Build history of the part. All positions in model axes, mm. A direction names the side the tool comes from. Give positions to 0.01 mm unless a question says otherwise; leave off trailing zeros. Return JSON: item names as keys, results as strings. Group by question number.
1) 3-axis set-ups, long thin cutter, end or side, ignore diameter. For faces 1 (the face through (-107.485, -173, 64)), 2 (the face through (-105.685, -173, 64)): which of +Z, -Z, +X, -X, +Y, -Y reach the whole face in a straight line?
2) Drop flat-ended pins along their axis: pin 1 (3 mm diameter, centred on y = -57, z = 57.5, fed in from +X); pin 2 (3 mm diameter, centred on y = -196, z = 73.5, fed in from +X); pin 3 (4.5 mm diameter, centred on y = -129, z = 53.5, fed in from +X). Give the stop position or say it passes through.
3) Slice it at A-A (y = -67.5). Count the separate pieces of the cut face and the enclosed holes in it, and give its area (3 significant figures).
4) Drill centre lines: probe 1 along Z at (x, y) = (-99, -293); probe 2 along Z at (x, y) = (-104.5, -229); probe 3 along X at (y, z) = (-174.5, 78.5). Where is each one in solid material? Low to high. Write a range as from..to.
5) Mould opens along X. For faces 3 (the face through (-87.485, -173, 64)), 4 (the face through (-102, -350, 69)), 5 (the face through (-89.285, -173, 64)) say: released by +X, released by -X, zero draft, split by the parting line, or undercut.
```python
from build123d import *

# Parameters (mm, degrees)
F0_R     = 2.5
F1_DEPTH = 350


with BuildPart() as f1:
    # F0 (on Front) → F1 (new body)
    with BuildSketch(Plane.XZ):
        with BuildLine():
            Line((-91.984542, 44.065978), (-88.984542, 44.065978))
            ThreePointArc((-88.984542, 44.065978), (-87.923881, 44.505318), (-87.484542, 45.565978))
            Line((-87.484542, 45.565978), (-87.484542, 48.565978))
            Line((-87.484542, 48.565978), (-87.484542, 50.465978))
            Line((-87.484542, 50.465978), (-87.784542, 50.465978))
            ThreePointArc((-87.784542, 50.465978), (-87.925963, 50.524557), (-87.984542, 50.665978))
            Line((-87.984542, 50.665978), (-87.984542, 50.965978))
            Line((-87.984542, 50.965978), (-89.284542, 50.965978))
            Line((-89.284542, 50.965978), (-89.284542, 48.565978))
            Line((-89.284542, 48.565978), (-90.923881, 48.565978))
            Line((-90.923881, 48.565978), (-92.998755, 50.640852))
            ThreePointArc((-92.998755, 50.640852), (-93.432301, 51.289698), (-93.584542, 52.055065))
            Line((-93.584542, 52.055065), (-93.584542, 56.076891))
            ThreePointArc((-93.584542, 56.076891), (-93.432301, 56.842257), (-92.998755, 57.491104))
            Line((-92.998755, 57.491104), (-90.923881, 59.565978))
            Line((-90.923881, 59.565978), (-89.284542, 59.565978))
            Line((-89.284542, 59.565978), (-89.284542, 57.165978))
            Line((-89.284542, 57.165978), (-87.984542, 57.165978))
            Line((-87.984542, 57.165978), (-87.984542, 57.465978))
            ThreePointArc((-87.984542, 57.465978), (-87.925963, 57.607399), (-87.784542, 57.665978))
            Line((-87.784542, 57.665978), (-87.484542, 57.665978))
            Line((-87.484542, 57.665978), (-87.484542, 59.565978))
            Line((-87.484542, 59.565978), (-87.484542, 62.565978))
            Line((-87.484542, 62.565978), (-87.484542, 64.065978))
            Line((-87.484542, 64.065978), (-87.484542, 65.565978))
            Line((-87.484542, 65.565978), (-87.484542, 68.565978))
            Line((-87.484542, 68.565978), (-87.484542, 70.465978))
            Line((-87.484542, 70.465978), (-87.784542, 70.465978))
            ThreePointArc((-87.784542, 70.465978), (-87.925963, 70.524557), (-87.984542, 70.665978))
            Line((-87.984542, 70.665978), (-87.984542, 70.965978))
            Line((-87.984542, 70.965978), (-89.284542, 70.965978))
            Line((-89.284542, 70.965978), (-89.284542, 68.565978))
            Line((-89.284542, 68.565978), (-90.923881, 68.565978))
            Line((-90.923881, 68.565978), (-92.998755, 70.640852))
            ThreePointArc((-92.998755, 70.640852), (-93.432301, 71.289698), (-93.584542, 72.055065))
            Line((-93.584542, 72.055065), (-93.584542, 76.076891))
            ThreePointArc((-93.584542, 76.076891), (-93.432301, 76.842257), (-92.998755, 77.491104))
            Line((-92.998755, 77.491104), (-90.923881, 79.565978))
            Line((-90.923881, 79.565978), (-89.284542, 79.565978))
            Line((-89.284542, 79.565978), (-89.284542, 77.165978))
            Line((-89.284542, 77.165978), (-87.984542, 77.165978))
            Line((-87.984542, 77.165978), (-87.984542, 77.465978))
            ThreePointArc((-87.984542, 77.465978), (-87.925963, 77.607399), (-87.784542, 77.665978))
            Line((-87.784542, 77.665978), (-87.484542, 77.665978))
            Line((-87.484542, 77.665978), (-87.484542, 79.565978))
            Line((-87.484542, 79.565978), (-87.484542, 82.565978))
            ThreePointArc((-87.484542, 82.565978), (-87.923881, 83.626638), (-88.984542, 84.065978))
            Line((-88.984542, 84.065978), (-91.984542, 84.065978))
            Line((-91.984542, 84.065978), (-93.384542, 84.065978))
            Line((-93.384542, 84.065978), (-93.884542, 84.065978))
            Line((-93.884542, 84.065978), (-93.884542, 83.765978))
            ThreePointArc((-93.884542, 83.765978), (-93.94312, 83.624557), (-94.084542, 83.565978))
            Line((-94.084542, 83.565978), (-94.384542, 83.565978))
            Line((-94.384542, 83.565978), (-94.384542, 82.265978))
            Line((-94.384542, 82.265978), (-91.984542, 82.265978))
            Line((-91.984542, 82.265978), (-91.984542, 80.626638))
            Line((-91.984542, 80.626638), (-94.059415, 78.551764))
            ThreePointArc((-94.059415, 78.551764), (-94.708262, 78.118219), (-95.473629, 77.965978))
            Line((-95.473629, 77.965978), (-99.495454, 77.965978))
            ThreePointArc((-99.495454, 77.965978), (-100.260821, 78.118219), (-100.909668, 78.551764))
            Line((-100.909668, 78.551764), (-102.984542, 80.626638))
            Line((-102.984542, 80.626638), (-102.984542, 82.265978))
            Line((-102.984542, 82.265978), (-100.584542, 82.265978))
            Line((-100.584542, 82.265978), (-100.584542, 83.565978))
            Line((-100.584542, 83.565978), (-100.884542, 83.565978))
            ThreePointArc((-100.884542, 83.565978), (-101.025963, 83.624557), (-101.084542, 83.765978))
            Line((-101.084542, 83.765978), (-101.084542, 84.065978))
            Line((-101.084542, 84.065978), (-101.584542, 84.065978))
            Line((-101.584542, 84.065978), (-102.984542, 84.065978))
            Line((-102.984542, 84.065978), (-105.984542, 84.065978))
            ThreePointArc((-105.984542, 84.065978), (-107.045202, 83.626638), (-107.484542, 82.565978))
            Line((-107.484542, 82.565978), (-107.484542, 79.565978))
            Line((-107.484542, 79.565978), (-107.484542, 77.665978))
            Line((-107.484542, 77.665978), (-107.184542, 77.665978))
            ThreePointArc((-107.184542, 77.665978), (-107.04312, 77.607399), (-106.984542, 77.465978))
            Line((-106.984542, 77.465978), (-106.984542, 77.165978))
            Line((-106.984542, 77.165978), (-105.684542, 77.165978))
            Line((-105.684542, 77.165978), (-105.684542, 79.565978))
            Line((-105.684542, 79.565978), (-104.045202, 79.565978))
            Line((-104.045202, 79.565978), (-101.970328, 77.491104))
            ThreePointArc((-101.970328, 77.491104), (-101.536782, 76.842257), (-101.384542, 76.076891))
            Line((-101.384542, 76.076891), (-101.384542, 72.055065))
            ThreePointArc((-101.384542, 72.055065), (-101.536782, 71.289698), (-101.970328, 70.640852))
            Line((-101.970328, 70.640852), (-104.045202, 68.565978))
            Line((-104.045202, 68.565978), (-105.684542, 68.565978))
            Line((-105.684542, 68.565978), (-105.684542, 70.965978))
            Line((-105.684542, 70.965978), (-106.984542, 70.965978))
            Line((-106.984542, 70.965978), (-106.984542, 70.665978))
            ThreePointArc((-106.984542, 70.665978), (-107.04312, 70.524557), (-107.184542, 70.465978))
            Line((-107.184542, 70.465978), (-107.484542, 70.465978))
            Line((-107.484542, 70.465978), (-107.484542, 68.565978))
            Line((-107.484542, 68.565978), (-107.484542, 65.565978))
            Line((-107.484542, 65.565978), (-107.484542, 64.065978))
            Line((-107.484542, 64.065978), (-107.484542, 62.565978))
            Line((-107.484542, 62.565978), (-107.484542, 59.565978))
            Line((-107.484542, 59.565978), (-107.484542, 57.665978))
            Line((-107.484542, 57.665978), (-107.184542, 57.665978))
            ThreePointArc((-107.184542, 57.665978), (-107.04312, 57.607399), (-106.984542, 57.465978))
            Line((-106.984542, 57.465978), (-106.984542, 57.165978))
            Line((-106.984542, 57.165978), (-105.684542, 57.165978))
            Line((-105.684542, 57.165978), (-105.684542, 59.565978))
            Line((-105.684542, 59.565978), (-104.045202, 59.565978))
            Line((-104.045202, 59.565978), (-101.970328, 57.491104))
            ThreePointArc((-101.970328, 57.491104), (-101.536782, 56.842257), (-101.384542, 56.076891))
            Line((-101.384542, 56.076891), (-101.384542, 52.055065))
            ThreePointArc((-101.384542, 52.055065), (-101.536782, 51.289698), (-101.970328, 50.640852))
            Line((-101.970328, 50.640852), (-104.045202, 48.565978))
            Line((-104.045202, 48.565978), (-105.684542, 48.565978))
            Line((-105.684542, 48.565978), (-105.684542, 50.965978))
            Line((-105.684542, 50.965978), (-106.984542, 50.965978))
            Line((-106.984542, 50.965978), (-106.984542, 50.665978))
            ThreePointArc((-106.984542, 50.665978), (-107.04312, 50.524557), (-107.184542, 50.465978))
            Line((-107.184542, 50.465978), (-107.484542, 50.465978))
            Line((-107.484542, 50.465978), (-107.484542, 48.565978))
            Line((-107.484542, 48.565978), (-107.484542, 45.565978))
            ThreePointArc((-107.484542, 45.565978), (-107.045202, 44.505318), (-105.984542, 44.065978))
            Line((-105.984542, 44.065978), (-102.984542, 44.065978))
            Line((-102.984542, 44.065978), (-101.584542, 44.065978))
            Line((-101.584542, 44.065978), (-101.084542, 44.065978))
            Line((-101.084542, 44.065978), (-101.084542, 44.365978))
            ThreePointArc((-101.084542, 44.365978), (-101.025963, 44.507399), (-100.884542, 44.565978))
            Line((-100.884542, 44.565978), (-100.584542, 44.565978))
            Line((-100.584542, 44.565978), (-100.584542, 45.865978))
            Line((-100.584542, 45.865978), (-102.984542, 45.865978))
            Line((-102.984542, 45.865978), (-102.984542, 47.505318))
            Line((-102.984542, 47.505318), (-100.909668, 49.580191))
            ThreePointArc((-100.909668, 49.580191), (-100.260821, 50.013737), (-99.495454, 50.165978))
            Line((-99.495454, 50.165978), (-95.473629, 50.165978))
            ThreePointArc((-95.473629, 50.165978), (-94.708262, 50.013737), (-94.059415, 49.580191))
            Line((-94.059415, 49.580191), (-91.984542, 47.505318))
            Line((-91.984542, 47.505318), (-91.984542, 45.865978))
            Line((-91.984542, 45.865978), (-94.384542, 45.865978))
            Line((-94.384542, 45.865978), (-94.384542, 44.565978))
            Line((-94.384542, 44.565978), (-94.084542, 44.565978))
            ThreePointArc((-94.084542, 44.565978), (-93.94312, 44.507399), (-93.884542, 44.365978))
            Line((-93.884542, 44.365978), (-93.884542, 44.065978))
            Line((-93.884542, 44.065978), (-93.384542, 44.065978))
            Line((-93.384542, 44.065978), (-91.984542, 44.065978))
        make_face()
        with Locations((-97.484542, 54.065978)):
            Circle(F0_R, mode=Mode.SUBTRACT)
        with BuildLine():
            ThreePointArc((-94.059415, 58.551764), (-94.708262, 58.118219), (-95.473629, 57.965978))
            Line((-95.473629, 57.965978), (-99.495454, 57.965978))
            ThreePointArc((-99.495454, 57.965978), (-100.260821, 58.118219), (-100.909668, 58.551764))
            Line((-100.909668, 58.551764), (-102.984542, 60.626638))
            Line((-102.984542, 60.626638), (-105.684542, 60.626638))
            Line((-105.684542, 60.626638), (-105.684542, 64.065978))
            Line((-105.684542, 64.065978), (-105.684542, 67.505318))
            Line((-105.684542, 67.505318), (-102.984542, 67.505318))
            Line((-102.984542, 67.505318), (-100.909668, 69.580191))
            ThreePointArc((-100.909668, 69.580191), (-100.260821, 70.013737), (-99.495454, 70.165978))
            Line((-99.495454, 70.165978), (-95.473629, 70.165978))
            ThreePointArc((-95.473629, 70.165978), (-94.708262, 70.013737), (-94.059415, 69.580191))
            Line((-94.059415, 69.580191), (-91.984542, 67.505318))
            Line((-91.984542, 67.505318), (-89.284542, 67.505318))
            Line((-89.284542, 67.505318), (-89.284542, 64.065978))
            Line((-89.284542, 64.065978), (-89.284542, 60.626638))
            Line((-89.284542, 60.626638), (-91.984542, 60.626638))
            Line((-91.984542, 60.626638), (-94.059415, 58.551764))
        make_face(mode=Mode.SUBTRACT)
        with Locations((-97.484542, 74.065978)):
            Circle(F0_R, mode=Mode.SUBTRACT)
    extrude(amount=F1_DEPTH)


solid = f1.part
```
Results:
{
 "1": {"face 1": "+Z, -Z, -X, +Y, -Y", "face 2": "+Y, -Y"},
 "2": {"pin 1": "x = -87.48", "pin 2": "x = -93.58", "pin 3": "x = -93.42"},
 "3": {"separate pieces": "1", "enclosed holes": "3", "area": "292 mm2"},
 "4": {"probe 1": "50.17..52.08, 56.05..57.97, 70.17..72.08, 76.05..77.97", "probe 2": "44.07..48.57, 59.57..60.63, 67.51..68.57, 79.57..84.07", "probe 3": "-107.48..-105.68, -102.98..-100.86, -94.11..-91.99, -89.28..-87.48"},
 "5": {"face 3": "released by +X", "face 4": "zero draft", "face 5": "undercut"}
}
